Model file for the job. Use its own axes, mm. Face numbers are marked on the shaded views. Round coordinates to 2 decimals unless told otherwise and drop trailing zeros. Loops run counter-clockwise (first coordinate to the right, second up) from the corner with the lowest first, then second, coordinate; pieces in that order, holes last. Notation, with made-up numbers: (53, -18) - (63, -18) arc R7 ccw to (63, -11) - close; hole circle Ø1 at (52, 21.25). An arc over 180 degrees is marked (long way). Use one line per item in the form item = value.
from build123d import *

# Parameters (mm, degrees)
SKETCH1_R            = 10
BOSS_EXTRUDE1_DEPTH  = 40
SKETCH2_R            = 20
BOSS_EXTRUDE2_DEPTH  = 10
FILLET1_R            = 10
FILLET1_OF_MIRROR1_R = 10


with BuildPart() as part:
    # Sketch1 → Boss-Extrude1 (new body)
    with BuildSketch(Plane(origin=(0, 0, 0), x_dir=(0, 0, -1), z_dir=(1, 0, 0))):
        Circle(SKETCH1_R)
    extrude(amount=BOSS_EXTRUDE1_DEPTH)

    # Sketch2 → Boss-Extrude2 (add)
    with BuildSketch(Plane(origin=(40, 0, 0), x_dir=(0, 0, -1), z_dir=(1, 0, 0))):
        Circle(SKETCH2_R)
    boss_extrude2 = extrude(amount=BOSS_EXTRUDE2_DEPTH)

    # Fillet1
    fillet1_edges = [part.edges().sort_by_distance(p)[0] for p in [
        (50, 0, 20),
    ]]
    fillet(fillet1_edges, radius=FILLET1_R - 0.0001)  # a hair under: the kernel refuses the full size

    # Mirror1: Boss-Extrude2 across plane
    add(boss_extrude2.mirror(Plane.ZY.offset(-20)))

    # Fillet1 of Mirror1
    fillet1_of_mirror1_edges = [part.edges().sort_by_distance(p)[0] for p in [
        (-10, 0, 20),
    ]]
    fillet(fillet1_of_mirror1_edges, radius=FILLET1_OF_MIRROR1_R - 0.0001)  # a hair under: the kernel refuses the full size


solid = part.part
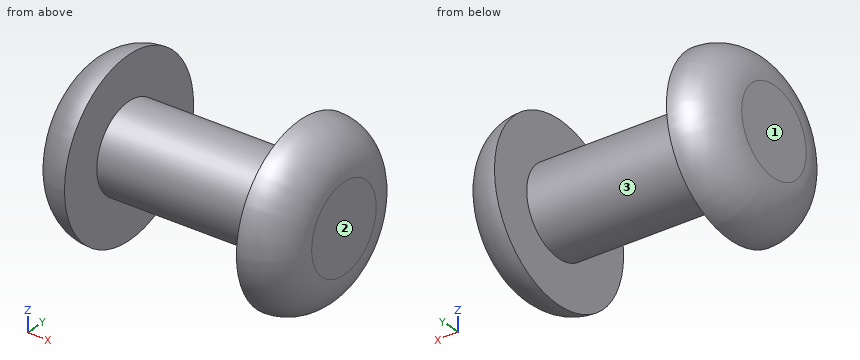
1. Cut at C-C, the plane x = 25.5. Give the cut face in (y, z), plus the area to 3 significant figures.
Geometry check:
outline = circle Ø20 at (0, 0)
area = 314 mm^2
2. Flat gauge pins, fed straight in: pin 1 (6 mm diameter, centred on x = 6.5, y = 5.5, fed in from -Z); pin 2 (4 mm diameter, centred on x = 5.5, z = -5, fed in from -Y); pin 3 (6 mm diameter, centred on x = 35.5, z = 8, fed in from -Y). Where does each tip first touch, or does it go through?
Geometry check:
pin_1 = -9.68
pin_2 = -9.54
pin_3 = -8.66
3. Wall check: probe 1 along X at (y, z) = (2.5, 15.5); probe 2 along X at (y, z) = (-0.5, 16.5); probe 3 along Y at (x, z) = (15, 0.5). Give the ranges that are in metal, low to high.
Geometry check:
probe_1 = -8.22 to 0, 40 to 48.22
probe_2 = -7.59 to 0, 40 to 47.59
probe_3 = -9.99 to 9.99
4. Pull direction X, two halves, no side cores. Call the marked faces 1, 2 and 3: +X half, -X half, draft (parallel to the pull), parting line (faces both ways), or undercut.
Geometry check:
face_1 = -X half
face_2 = +X half
face_3 = undercut
5. Cut at D-D, the plane x = 42. Give the cut face in (y, z).
Geometry check:
outline = circle Ø39.6 at (0, 0)
